Build history of the part. All positions in model axes, mm. A direction names the side the tool comes from. Round coordinates to 2 decimals unless told otherwise and drop trailing zeros. Write each loop counter-clockwise with the first axis right and the second up, starting at its lowest first coordinate (ties: lowest second). Pieces come first, ordered by that corner, then holes. Notation, with made-up numbers: (-2, 8) -> (34, 8) arc R26 cw to (34, 44) -> close; hole circle Ø2 at (86.5, 30). An arc over 180 degrees is marked (long way). Answer in a Markdown table with one row per item.
```python
from build123d import *

# Parameters (mm, degrees)
F0_W     = 88.9
F0_H     = 165.1
F1_DEPTH = 6.35
F2_DEPTH = 25.4
F3_DEPTH = 50.8
F4_R     = 5.08
F5_SIZE2 = 7.3323484187
F5_SIZE  = 12.7
F6_SIZE2 = 7.3323484187
F6_SIZE  = 12.7
F7_SIZE2 = 7.3323484187
F7_SIZE  = 12.7


with BuildPart() as f1:
    # F0 (on Top) → F1 (new body)
    with BuildSketch(Plane.XY):
        with Locations((5.6305658072, 24.3604830414)):
            Rectangle(F0_W, F0_H)
        Polygon((-32.4694341928, 56.1104830414), (-32.4694341928, 100.5604830414), (5.6305658072, 100.5604830414), (43.7305658072, 100.5604830414), (43.7305658072, -13.7395169586), (43.7305658072, -51.8395169586), (5.6305658072, -51.8395169586), (-32.4694341928, -51.8395169586), align=None, mode=Mode.SUBTRACT)
    extrude(amount=F1_DEPTH)

    # F0 (on Top) → F2 (join)
    with BuildSketch(Plane.XY):
        with BuildLine():
            Line((43.7305658072, 100.5604830414), (5.6305658072, 100.5604830414))
            Line((5.6305658072, 100.5604830414), (5.6305658072, 68.8104830414))
            ThreePointArc((5.6305658072, 68.8104830414), (1.9108219283, 59.8302269203), (-7.0694341928, 56.1104830414))
            Line((-7.0694341928, 56.1104830414), (-32.4694341928, 56.1104830414))
            Line((-32.4694341928, 56.1104830414), (-32.4694341928, -51.8395169586))
            Line((-32.4694341928, -51.8395169586), (5.6305658072, -51.8395169586))
            Line((5.6305658072, -51.8395169586), (5.6305658072, -26.4395169586))
            ThreePointArc((5.6305658072, -26.4395169586), (9.3503096862, -17.4592608375), (18.3305658072, -13.7395169586))
            Line((18.3305658072, -13.7395169586), (43.7305658072, -13.7395169586))
            Line((43.7305658072, -13.7395169586), (43.7305658072, 100.5604830414))
        make_face()
    extrude(amount=F2_DEPTH)

    # F0 (on Top) → F3 (join)
    with BuildSketch(Plane.XY):
        with BuildLine():
            Line((43.7305658072, -51.8395169586), (43.7305658072, -13.7395169586))
            Line((43.7305658072, -13.7395169586), (18.3305658072, -13.7395169586))
            ThreePointArc((18.3305658072, -13.7395169586), (9.3503096862, -17.4592608375), (5.6305658072, -26.4395169586))
            Line((5.6305658072, -26.4395169586), (5.6305658072, -51.8395169586))
            Line((5.6305658072, -51.8395169586), (43.7305658072, -51.8395169586))
        make_face()
        with BuildLine():
            Line((5.6305658072, 100.5604830414), (-32.4694341928, 100.5604830414))
            Line((-32.4694341928, 100.5604830414), (-32.4694341928, 56.1104830414))
            Line((-32.4694341928, 56.1104830414), (-7.0694341928, 56.1104830414))
            ThreePointArc((-7.0694341928, 56.1104830414), (1.9108219283, 59.8302269203), (5.6305658072, 68.8104830414))
            Line((5.6305658072, 68.8104830414), (5.6305658072, 100.5604830414))
        make_face()
    extrude(amount=F3_DEPTH)

    # F4
    f4_edges = [f1.edges().sort_by_distance(p)[0] for p in [
        (-38.819434, 24.360483, 6.35),
        (5.630566, -58.189517, 6.35),
        (50.080566, 24.360483, 6.35),
        (5.630566, 106.910483, 6.35),
    ]]
    fillet(f4_edges, radius=F4_R)

    # F5
    f5_edges = [f1.edges().sort_by_distance(p)[0] for p in [
        (43.730566, 43.410483, 25.4),
        (24.680566, 100.560483, 25.4),
        (-32.469434, 2.135483, 25.4),
        (-13.419434, -51.839517, 25.4),
    ]]
    chamfer(f5_edges, length=F5_SIZE, length2=F5_SIZE2)

    # F6
    f6_edges = [f1.edges().sort_by_distance(p)[0] for p in [
        (24.680566, -51.839517, 50.8),
        (43.730566, -32.789517, 50.8),
    ]]
    f6_side = f1.faces().sort_by_distance((25.076608, -33.185559, 50.8))[0]
    chamfer(f6_edges, length=F6_SIZE, length2=F6_SIZE2, reference=f6_side)

    # F7
    f7_edges = [f1.edges().sort_by_distance(p)[0] for p in [
        (-32.469434, 78.335483, 50.8),
        (-13.419434, 100.560483, 50.8),
    ]]
    f7_side = f1.faces().sort_by_distance((-13.757718, 78.740013, 50.8))[0]
    chamfer(f7_edges, length=F7_SIZE, length2=F7_SIZE2, reference=f7_side)


solid = f1.part
```
Q1. Saw through at B-B on y = -32. Write the cut outline in (x, z).
A:
| item | result |
|---|---|
| outline | (-38.82, 0) -> (50.08, 0) -> (50.08, 1.27) arc R5.08 ccw to (45, 6.35) -> (43.73, 6.35) -> (43.73, 43.47) -> (31.03, 50.8) -> (5.63, 50.8) -> (5.63, 25.4) -> (-25.14, 25.4) -> (-32.47, 12.7) -> (-32.47, 6.35) -> (-33.74, 6.35) arc R5.08 ccw to (-38.82, 1.27) -> close |
Q2. Which spindle directions (+Z, -Z, +X, -X, +Y, -Y) get a long thin tool onto all of the face, cutting with end or side? Do faces 1 (the flat face through (37.47, -28.82, 47.08)), 2 (the flat face through (40.013, 42.61, 19.139)), 3 (the flat face through (20.18, -45.58, 47.08)), 4 (the flat face through (-11, 100.56, 21)), 5 (the flat face through (-13.69, -48.12, 19.14)). Say none if no direction does.
A:
| item | result |
|---|---|
| face 1 | +Z, +X, +Y, -Y |
| face 2 | +Z, +X, +Y |
| face 3 | +Z, +X, -X, -Y |
| face 4 | +Z, +X, -X, +Y |
| face 5 | +Z, -X, -Y |
Q3. Saw through at C-C on x = -22.5. Write the cut outline in (y, z), plus the area to 3 significant figures.
A:
| item | result |
|---|---|
| outline | (-58.19, 0) -> (106.91, 0) -> (106.91, 1.27) arc R5.08 ccw to (101.83, 6.35) -> (100.56, 6.35) -> (100.56, 43.47) -> (90.59, 49.22) -> (56.11, 49.22) -> (56.11, 25.4) -> (-44.51, 25.4) -> (-51.84, 12.7) -> (-51.84, 6.35) -> (-53.11, 6.35) arc R5.08 ccw to (-58.19, 1.27) -> close |
| area | 4,920 mm² |
Q4. Saw through at D-D on z = 16.5. Write the cut outline in (x, y), plus the area to 3 significant figures.
A:
| item | result |
|---|---|
| outline | (-32.47, 56.11) -> (-30.28, 56.11) -> (-30.28, -49.65) -> (5.63, -49.65) -> (5.63, -51.84) -> (43.73, -51.84) -> (43.73, -13.74) -> (41.54, -13.74) -> (41.54, 98.37) -> (5.63, 98.37) -> (5.63, 100.56) -> (-32.47, 100.56) -> close |
| area | 11,000 mm² |
Q5. Drop flat-ended pins along their axis: P1, Ø5, axis at x = 25, y = 71.5, coming from the +Z side; P2, Ø1, axis at x = -16, z = 17.5, coming from the -Y side; P3, Ø2, axis at x = 15, z = 37.5, coming from the +Y side. Give the stop position or say it passes through.
A:
| item | result |
|---|---|
| P1 | z = 25.4 |
| P2 | y = -49.36 |
| P3 | y = -13.96 |
Q6. Wall check: line 1 (X direction, y = 15, z = 7); line 2 (Y direction, x = 34, z = 33); line 3 (Z direction, x = 7.5, y = 18). Give the ranges that are in metal, low to high. Write a range as [from, to].
A:
| item | result |
|---|---|
| line 1 | [-32.47, 43.73] |
| line 2 | [-51.84, -13.74] |
| line 3 | [0, 25.4] |
Q7. Two-plate mould, pull along Z, no slides. Class faces 6 (the flat face through (5, 25, 25.4)), 7 (the flat face through (22, -51.84, 21)): released by +Z, released by -Z, zero draft, split by the parting line, or undercut.
A:
| item | result |
|---|---|
| face 6 | released by +Z |
| face 7 | zero draft |
Q8. Saw through at A-A on z = 27. Write the cut outline in (x, y), plus the area to 3 significant figures.
A:
| item | result |
|---|---|
| outline | (-32.47, 56.11) -> (-7.07, 56.11) arc R12.7 ccw to (5.63, 68.81) -> (5.63, 100.56) -> (-32.47, 100.56) -> close; (5.63, -51.84) -> (43.73, -51.84) -> (43.73, -13.74) -> (18.33, -13.74) arc R12.7 ccw to (5.63, -26.44) -> close |
| area | 3,080 mm² |
